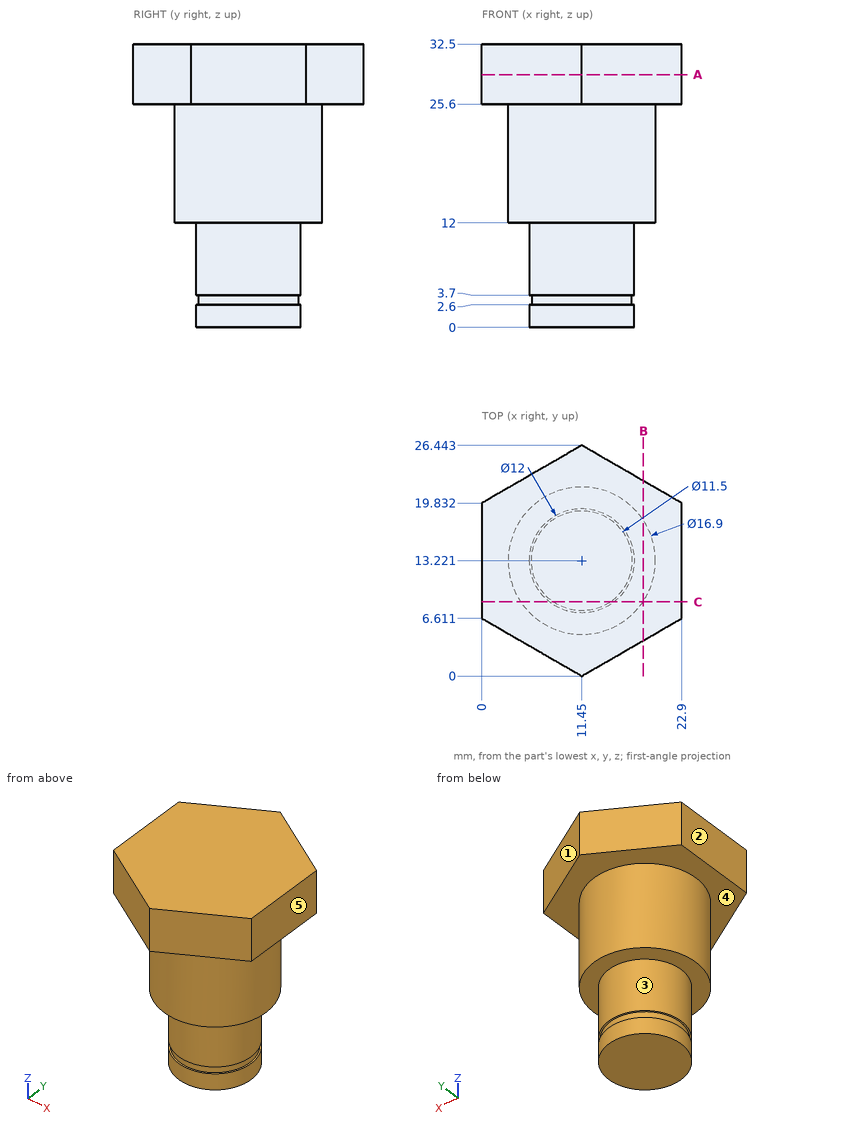
Check sheet for the drawn part. Datum: minimum x, y, z corner. Units: mm. A direction names the side the tool comes from. Coordinates: 2 decimals unless noted, no trailing zeros. Order: outer loops, then holes, each group sorted by start corner. A loop starts at its lowest first (then second) coordinate and runs counter-clockwise, first axis right, second up. Notation, with made-up numbers: M 10.5,-11.75 L 34.5,-11.75 A16 ccw 34.5,15.25 Z; hole C 45.25,-2.75 d6. An arc over 180 degrees is marked long. One line per item, written item: value. Start each with the question number.
Item 1: Sectioned sample at C-C (y = 8.5). Enter the section's corners in (x, z).
Item 2: Mould release check, pull along Y, two halves, no side actions. Record for the marked faces 1, 2 and 3: released by +Y, released by -Y, zero draft, split by the parting line, or undercut.
Item 3: Access from +Z, -Z, +X, -X, +Y, -Y to the whole of each face (thin tool, end or side, straight path). Record for the marked faces 4 and 5.
Item 4: Sectioned sample at A-A (z = 29). Enter the section's corners in (x, y).
Item 5: Gauge pin test, flat ends, axial feed: pin 1 (10 mm diameter, centred on x = 6.5, z = 29, fed in from +Y); pin 2 (4 mm diameter, centred on y = 13.5, z = 11.5, fed in from +X); pin 3 (3 mm diameter, centred on x = 20, z = 26.5, fed in from +Y). Record the tip position at first contact, or that the pin passes through.
Item 6: Sectioned sample at B-B (x = 18.5). Enter the section's corners in (y, z), then the cut area to 3 significant figures.
Item 7: Scan lines: probe 1 along Z at (x, y) = (12, 20.25); probe 2 along Y at (x, z) = (5.5, 19.5); probe 3 along Y at (x, z) = (6.75, 24) (1 decimal). Record each from-to range of solid material in increasing order.
Conclusion:
1. outline: M 0,25.6 L 4.44,25.6 L 4.44,12 L 7.75,12 L 7.75,3.7 L 8.17,3.7 L 8.17,2.6 L 7.75,2.6 L 7.75,0 L 15.15,0 L 15.15,2.6 L 14.73,2.6 L 14.73,3.7 L 15.15,3.7 L 15.15,12 L 18.46,12 L 18.46,25.6 L 22.9,25.6 L 22.9,32.5 L 0,32.5 Z
2. face 1: released by +Y
2. face 2: zero draft
2. face 3: split by the parting line
3. face 4: -Z
3. face 5: +Z, -Z, +X, +Y, -Y
4. outline: M 0,6.61 L 11.45,0 L 22.9,6.61 L 22.9,19.83 L 11.45,26.44 L 0,19.83 Z
5. pin 1: stops at y = 26.44
5. pin 2: stops at x = 19.9
5. pin 3: stops at y = 22.37
6. outline: M 4.07,25.6 L 8.56,25.6 L 8.56,12 L 17.88,12 L 17.88,25.6 L 22.37,25.6 L 22.37,32.5 L 4.07,32.5 Z
6. area: 253 mm^2
7. probe 1: z = 12 to 32.5
7. probe 2: y = 7.22 to 19.22
7. probe 3: y = 6.2 to 20.2
